The model under review builds one solid part; all positions refer to its coordinate system, in mm. A direction names the side the tool comes from. Round coordinates to 2 decimals unless told otherwise and drop trailing zeros. Write each loop counter-clockwise with the first axis right and the second up, starting at its lowest first coordinate (ties: lowest second). Pieces come first, ordered by that corner, then holes. Notation, with made-up numbers: (10.5, 74) - (63.5, 74) arc R24 cw to (63.5, 108) - close; hole circle Ø7 at (89, 46). An arc over 180 degrees is marked (long way). Write each question's results on one line, items separated by ' | '.
```python
from build123d import *

# Parameters (mm, degrees)
SKETCH1_R                 = 330.2
BOSS_EXTRUDE1_DEPTH       = 55
SKETCH2_R                 = 330.2
BOSS_EXTRUDE2_DEPTH       = 55
BOSS_EXTRUDE3_DEPTH       = 10
BOSS_EXTRUDE6_DEPTH       = 575.8
BOSS_EXTRUDE33_DEPTH      = 370
BOSS_EXTRUDE33_DEPTH_BACK = 370
SKETCH25_W                = 366.7
SKETCH25_H                = 80
SKETCH5_W                 = 450
SKETCH5_H                 = 72
BOSS_EXTRUDE7_DEPTH       = 367.981167426
SKETCH8_W                 = 49.2
SKETCH8_H                 = 29.2
BOSS_EXTRUDE13_DEPTH      = 30
SKETCH19_R                = 177.8
BOSS_EXTRUDE22_DEPTH      = 270.2
CHAMFER1_SIZE             = 100
CHAMFER1_SIZE2            = 93.251508614
BOSS_EXTRUDE27_DEPTH      = 30
BOSS_EXTRUDE20_DEPTH      = 260
SKETCH23_W                = 30
SKETCH23_H                = 60
SKETCH23_W_2              = 49.2
SKETCH23_H_2              = 25.4
SKETCH23_W_3              = 25.4
BOSS_EXTRUDE28_DEPTH      = 30
SKETCH24_R                = 177.8
BOSS_EXTRUDE29_DEPTH      = 270.2
CHAMFER2_SIZE             = 100
CHAMFER2_SIZE2            = 93.251508614
BOSS_EXTRUDE30_DEPTH      = 30
BOSS_EXTRUDE31_DEPTH      = 260
SKETCH16_W                = 250
SKETCH16_H                = 53.975
BOSS_EXTRUDE18_DEPTH      = 53.975
SKETCH18_W                = 250
SKETCH18_H                = 53.975
BOSS_EXTRUDE19_DEPTH      = 53.975
BOSS_EXTRUDE32_REACH      = 1866.083
BOSS_EXTRUDE34_REACH      = 1575.824
SKETCH26_W                = 154.1
SKETCH26_H                = 80
SKETCH27_W                = 350
SKETCH27_H                = 400
BOSS_EXTRUDE35_DEPTH      = 200
BOSS_EXTRUDE36_START      = -130
BOSS_EXTRUDE36_DEPTH      = 490
FILLET3_R                 = 50
SKETCH30_W                = 2623.123535912
SKETCH30_H                = 2390.43733062
CUT_EXTRUDE1_DEPTH        = 1887.551796433
SKETCH31_W                = 2584.765961417
SKETCH31_H                = 1828.147621016
CUT_EXTRUDE2_DEPTH        = 1855.050466041


with BuildPart() as part:
    # Sketch1 → Boss-Extrude1 (new body)
    with BuildSketch(Plane.XY):
        with Locations((330.2, 330.2)):
            Circle(SKETCH1_R)
    extrude(amount=-BOSS_EXTRUDE1_DEPTH)



with BuildPart() as body_2:
    # Sketch2 → Boss-Extrude2 (new body)
    with BuildSketch(Plane.XY.offset(-685.8)):
        with Locations((330.2, 330.2)):
            Circle(SKETCH2_R)
    extrude(amount=BOSS_EXTRUDE2_DEPTH)


with BuildPart() as part_1:
    add(part.part)

    add(body_2.part)  # Boss-Extrude3 merges body 2
    # 3DSketch2 → Boss-Extrude3 (add)
    with BuildSketch(Plane(origin=(330.2, 460, -630.8), x_dir=(0.5893057409504111, 0, 0.807910108664873), z_dir=(0, -1, 0))):
        Polygon((465.194640569, 339.322245639), (0, 0), (247.508411199, -339.322245639), (712.703051768, 0), align=None)
        Polygon((-38.304873162, 52.514157063), (0, 0), (465.194640569, 339.322245639), (426.889767407, 391.836402702), align=None)
    extrude(amount=-BOSS_EXTRUDE3_DEPTH)

    # Sketch4 → Boss-Extrude6 (add)
    with BuildSketch(Plane(origin=(0, -170.8, -630.8), x_dir=(1, 0, 0), z_dir=(0, 0, 1))):
        Polygon((208.828935151, 1364.6), (330.2, 501), (265.832575532, 491.953748438), (143.190142937, 1364.6), align=None)
    extrude(amount=BOSS_EXTRUDE6_DEPTH)

    # Sketch5 → Boss-Extrude7 (add, along a direction that is not the sketch's normal)
    with BuildSketch(Plane(origin=(0, 470, 0), x_dir=(1, 0, 0), z_dir=(0, 1, 0))):
        with Locations((535.552391309, 91)):
            Rectangle(SKETCH5_W, SKETCH5_H)
        with Locations((535.552391309, 594.8)):
            Rectangle(SKETCH5_W, SKETCH5_H)
    extrude(amount=BOSS_EXTRUDE7_DEPTH, dir=(-0.13917310096006222, 0.9902680687415708, 0))

    # Sketch8 → Boss-Extrude13 (add)
    with BuildSketch(Plane(origin=(0, 0, -630.8), x_dir=(-1, 0, 0), z_dir=(0, 0, -1))):
        Polygon((-1014.4, 360.2), (-939.8, 360.2), (-939.8, 330.2), (-914.4, 330.2), (-914.4, 270.2), (-884.4, 270.2), (-884.4, 330.2), (-330.2, 330.2), (-325.983774959, 360.2), (-914.4, 360.2), (-914.4, 414.8), (-884.4, 414.8), (-884.4, 440.2), (-1014.4, 440.2), align=None)
        with Locations((-964.4, 400.2)):
            Rectangle(SKETCH8_W, SKETCH8_H, mode=Mode.SUBTRACT)
    extrude(amount=-BOSS_EXTRUDE13_DEPTH)

    # Sketch19 → Boss-Extrude22 (add)
    with BuildSketch(Plane.XZ.offset(-270.2)):
        with Locations(Location((899.4, -615.8, 0), (0, 0, 90))):
            Circle(SKETCH19_R)
    extrude(amount=BOSS_EXTRUDE22_DEPTH)

    # Chamfer1
    chamfer1_edges = [part_1.edges().sort_by_distance(p)[0] for p in [
        (899.4, 270.2, -793.6),
    ]]
    chamfer1_side = [part_1.faces().sort_by_distance(p)[0] for p in [
        (899.4, 270.2, -788.571056572),
    ]]
    chamfer(chamfer1_edges, length=CHAMFER1_SIZE, length2=CHAMFER1_SIZE2, reference=chamfer1_side[0])

    # Sketch8<7> → Boss-Extrude27 (add)
    with BuildSketch(Plane(origin=(0, 0, -630.8), x_dir=(-1, 0, 0), z_dir=(0, 0, -1))):
        Polygon((-1014.4, 360.2), (-1140.7, 120.65), (-1115.3, 120.65), (-989, 360.2), align=None)
    extrude(amount=-BOSS_EXTRUDE27_DEPTH)

    # Sketch8<4> → Boss-Extrude20 (add)
    with BuildSketch(Plane(origin=(0, 0, -630.8), x_dir=(-1, 0, 0), z_dir=(0, 0, -1))):
        Polygon((-1226.425, 111.125), (-1226.425, 120.65), (-1140.7, 120.65), (-1115.3, 120.65), (-1029.575, 120.65), (-1029.575, 111.125), align=None)
    extrude(amount=-BOSS_EXTRUDE20_DEPTH)

    # Sketch23 → Boss-Extrude28 (add)
    with BuildSketch(Plane(origin=(0, 0, -55), x_dir=(-1, 0, 0), z_dir=(0, 0, -1))):
        with BuildLine():
            Line((-330.2, 360.2), (-659.034365601, 360.2))
            ThreePointArc((-659.034365601, 360.2), (-660.058414719, 345.215533268), (-660.4, 330.2))
            Line((-660.4, 330.2), (-330.2, 330.2))
            Line((-330.2, 330.2), (-330.2, 360.2))
        make_face()
        with BuildLine():
            Line((-914.4, 360.2), (-939.8, 360.2))
            Line((-939.8, 360.2), (-939.8, 330.2))
            Line((-939.8, 330.2), (-914.4, 330.2))
            Line((-914.4, 330.2), (-884.4, 330.2))
            Line((-884.4, 330.2), (-660.4, 330.2))
            ThreePointArc((-660.4, 330.2), (-660.058414719, 345.215533268), (-659.034365601, 360.2))
            Line((-659.034365601, 360.2), (-914.4, 360.2))
        make_face()
        with Locations((-899.4, 300.2)):
            Rectangle(SKETCH23_W, SKETCH23_H)
        Polygon((-939.8, 385.6), (-939.8, 360.2), (-914.4, 360.2), (-914.4, 414.8), (-914.4, 440.2), (-939.8, 440.2), (-939.8, 414.8), align=None)
        with Locations((-964.4, 372.9)):
            Rectangle(SKETCH23_W_2, SKETCH23_H_2)
        with Locations((-964.4, 427.5)):
            Rectangle(SKETCH23_W_2, SKETCH23_H_2)
        Polygon((-1014.4, 440.2), (-1014.4, 385.6), (-989, 385.6), (-989, 414.8), (-989, 440.2), align=None)
        with Locations((-1001.7, 372.9)):
            Rectangle(SKETCH23_W_3, SKETCH23_H_2)
        Polygon((-325.983774959, 360.2), (-330.2, 360.2), (-330.2, 330.2), align=None)
        with Locations((-899.4, 427.5)):
            Rectangle(SKETCH23_W, SKETCH23_H_2)
    extrude(amount=BOSS_EXTRUDE28_DEPTH)

    # Sketch24 → Boss-Extrude29 (add)
    with BuildSketch(Plane(origin=(0, 270.2, 0), x_dir=(-1, 0, 0), z_dir=(0, -1, 0))):
        with Locations(Location((-899.4, 70, 0), (0, 0, 270))):
            Circle(SKETCH24_R)
    extrude(amount=BOSS_EXTRUDE29_DEPTH)

    # Chamfer2
    chamfer2_edges = [part_1.edges().sort_by_distance(p)[0] for p in [
        (899.4, 270.2, -247.8),
    ]]
    chamfer2_side = [part_1.faces().sort_by_distance(p)[0] for p in [
        (899.4, 270.2, -242.771056572),
    ]]
    chamfer(chamfer2_edges, length=CHAMFER2_SIZE, length2=CHAMFER2_SIZE2, reference=chamfer2_side[0])

    # Sketch23<10> → Boss-Extrude30 (add)
    with BuildSketch(Plane(origin=(0, 0, -55), x_dir=(-1, 0, 0), z_dir=(0, 0, -1))):
        Polygon((-1014.4, 360.2), (-1140.7, 120.65), (-1115.3, 120.65), (-989, 360.2), align=None)
    extrude(amount=BOSS_EXTRUDE30_DEPTH)

    # Sketch23<12> → Boss-Extrude31 (add)
    with BuildSketch(Plane(origin=(0, 0, -55), x_dir=(-1, 0, 0), z_dir=(0, 0, -1))):
        Polygon((-1226.425, 111.125), (-1226.425, 120.65), (-1140.7, 120.65), (-1115.3, 120.65), (-1029.575, 120.65), (-1029.575, 111.125), align=None)
    extrude(amount=BOSS_EXTRUDE31_DEPTH)

    # Sketch16 → Boss-Extrude18 (add)
    with BuildSketch(Plane(origin=(0, 0, -630.8), x_dir=(-1, 0, 0), z_dir=(0, 0, -1))):
        with Locations((-58.349686454, 935.0375)):
            Rectangle(SKETCH16_W, SKETCH16_H)
    extrude(amount=-BOSS_EXTRUDE18_DEPTH)

    # Sketch18 → Boss-Extrude19 (add)
    with BuildSketch(Plane(origin=(0, 0, -55), x_dir=(-1, 0, 0), z_dir=(0, 0, -1))):
        with Locations((-58.349686454, 935.0375)):
            Rectangle(SKETCH18_W, SKETCH18_H)
    extrude(amount=BOSS_EXTRUDE19_DEPTH)

    # Boss-Extrude32: up to this face of the body (flat: up to its plane)
    boss_extrude32_end = Plane(part_1.part.faces().sort_by_distance((283.205191665, 255.458003874, -55))[0])
    # Sketch8<8> → Boss-Extrude32 (add, up to the picked face)
    with BuildSketch(Plane(origin=(0, 0, -630.8), x_dir=(-1, 0, 0), z_dir=(0, 0, -1)), mode=Mode.PRIVATE) as boss_extrude32_sk1:
        Polygon((-314.740508183, 440.2), (-283.793416381, 660.4), (-914.4, 660.4), (-914.4, 440.2), align=None)
    boss_extrude32_tool1 = split(extrude(boss_extrude32_sk1.sketch, amount=-BOSS_EXTRUDE32_REACH, mode=Mode.PRIVATE), bisect_by=boss_extrude32_end, keep=Keep.BOTH, mode=Mode.PRIVATE)
    add(boss_extrude32_tool1.solids().sort_by(Axis((606.768609, 551.223181, -630.8), (0, 0, 1)))[0])



with BuildPart() as body_2_2:
    # Sketch25 → Boss-Extrude33 (new, two sides: drawn at the far end of the back side and taken through both)
    with BuildSketch(Plane.XY.offset(-342.9).offset(-BOSS_EXTRUDE33_DEPTH_BACK)):
        with Locations((760.189311143, 874.4)):
            Rectangle(SKETCH25_W, SKETCH25_H)
    extrude(amount=BOSS_EXTRUDE33_DEPTH + BOSS_EXTRUDE33_DEPTH_BACK)


with BuildPart() as part_2:
    add(part_1.part)

    add(body_2_2.part)  # Boss-Extrude34 merges body 2 2
    # Boss-Extrude34: up to this plane
    boss_extrude34_end = Plane(origin=(143.190142937, 1193.8, 837.459616456), z_dir=(0.9902680687415708, 0.13917310096006216, 0))
    # Sketch26 → Boss-Extrude34 (add, up to the surface)
    with BuildSketch(Plane.ZY.offset(-576.839311143), mode=Mode.PRIVATE) as boss_extrude34_sk1:
        with Locations((-49.95, 874.4)):
            Rectangle(SKETCH26_W, SKETCH26_H)
    boss_extrude34_tool1 = split(extrude(boss_extrude34_sk1.sketch, amount=BOSS_EXTRUDE34_REACH, mode=Mode.PRIVATE), bisect_by=boss_extrude34_end, keep=Keep.BOTH, mode=Mode.PRIVATE)
    add(boss_extrude34_tool1.solids().sort_by_distance((576.839311, 874.4, -49.95))[0])
    # Sketch26 → Boss-Extrude34 (add, up to the surface)
    with BuildSketch(Plane.ZY.offset(-576.839311143), mode=Mode.PRIVATE) as boss_extrude34_sk2:
        with Locations((-635.85, 874.4)):
            Rectangle(SKETCH26_W, SKETCH26_H)
    boss_extrude34_tool2 = split(extrude(boss_extrude34_sk2.sketch, amount=BOSS_EXTRUDE34_REACH, mode=Mode.PRIVATE), bisect_by=boss_extrude34_end, keep=Keep.BOTH, mode=Mode.PRIVATE)
    add(boss_extrude34_tool2.solids().sort_by_distance((576.839311, 874.4, -635.85))[0])

    # Sketch27 → Boss-Extrude35 (add)
    with BuildSketch(Plane(origin=(304.944608977, 42.857169884, 0), x_dir=(0, 0, 1), z_dir=(-0.9902680687415708, -0.13917310096006216, 0))):
        with Locations((-342.9, 481.031558361)):
            Rectangle(SKETCH27_W, SKETCH27_H)
    extrude(amount=BOSS_EXTRUDE35_DEPTH)

    # Sketch29 → Boss-Extrude36 (add)
    with BuildSketch(Plane(origin=(0, 0, -712.9), x_dir=(-1, 0, 0), z_dir=(0, 0, -1)).offset(BOSS_EXTRUDE36_START)):
        Polygon((-1029.044346974, 1149.323155196), (-986.95135556, 1160.601938253), (-943.539311143, 914.4), align=None)
        Polygon((-986.95135556, 1160.601938253), (-943.539311143, 914.4), (-923.230778905, 914.4), (-967.2552005, 1164.074901806), align=None)
    extrude(amount=-BOSS_EXTRUDE36_DEPTH)

    # Fillet3
    fillet3_edges = [part_2.edges().sort_by_distance(p)[0] for p in [
        (914.4, 660.4, -342.9),
    ]]
    fillet(fillet3_edges, radius=FILLET3_R)

    # Sketch30 → Cut-Extrude1 (cut, through all)
    with BuildSketch(Plane.XY):
        with Locations((451.826678709, -534.81866531)):
            Rectangle(SKETCH30_W, SKETCH30_H)
    extrude(amount=CUT_EXTRUDE1_DEPTH, mode=Mode.SUBTRACT)

    # Sketch31 → Cut-Extrude2 (cut, through all)
    with BuildSketch(Plane(origin=(0, 0, -685.8), x_dir=(-1, 0, 0), z_dir=(0, 0, -1))):
        with Locations((-741.050727566, -253.673810508)):
            Rectangle(SKETCH31_W, SKETCH31_H)
    extrude(amount=CUT_EXTRUDE2_DEPTH, mode=Mode.SUBTRACT)


solid = part_2.part
```
Q1. The part is to be moulded in two halves that separate along Z. For faces 5 (the flat face through (964, 440.2, -616)), 6 (the flat face through (975, 1069, -582.9)), 7 (the flat face through (826, 340, -600.8)), say which applies: released by +Z, released by -Z, zero draft, split by the parting line, or undercut.
Evaluation:
face 5: zero draft | face 6: released by -Z | face 7: undercut
Q2. We need section B-B (y = 547). State the section outline as (x, z) points, plus the area to 3 significant figures.
Evaluation:
outline: (32.13, -517.9) - (234.09, -517.9) - (234.09, -630.8) - (81.14, -630.8) - (81.14, -685.8) - (579.26, -685.8) - (579.26, -630.8) - (914.4, -630.8) - (914.4, -55) - (579.26, -55) - (579.26, 0) - (81.14, 0) - (81.14, -55) - (234.09, -55) - (234.09, -167.9) - (32.13, -167.9) - close | area: 517,000 mm^2
Q3. Tool access review of faces 1 (the flat face through (914.4, 526, -347)), 2 (the flat face through (939.8, 345, -70)), 3 (the flat face through (60, 908.05, -82)), 4 (the flat face through (494, 786, -127)): name each direction out of +Z, -Z, +X, -X, +Y, -Y from which nothing blocks a thin tool from reaching the whole face with its end or side.
Evaluation:
face 1: +Z, -Z, +X | face 2: +Z, -Z | face 3: +Z, -Z, -X, -Y | face 4: none
Q4. Insertion check: P1, Ø4, axis at x = 256.5, y = 746.5, coming from the +Z side; P2, Ø9, axis at x = 627.5, z = -610.5, coming from the +Y side; P3, Ø15, axis at y = 340, z = -65.5, coming from the +X side. Each pin has a flat end and moves straight along its axis. Give the tip position at first contact, or say it passes through.
Evaluation:
P1: stops at z = -55 | P2: stops at y = 914.4 | P3: stops at x = 1029
Q5. For probe 1 along Y at (x, z) = (851.5, -609); probe 2 along Z at (x, y) = (197.5, 478); probe 3 along Y at (x, z) = (597, -513), list the stretches that pass through material, from the lowest coordinate up.
Evaluation:
probe 1: y = 0 to 270.2, 330.2 to 360.2, 440.2 to 660.4, 834.4 to 914.4 | probe 2: z = -685.8 to -630.8, -517.9 to -167.9, -55 to 0 | probe 3: y = 440.2 to 660.4, 834.4 to 914.4
Q6. We need section A-A (x = 451.5). State the section outline as (y, z) points.
Evaluation:
outline: (23.09, -685.8) - (637.31, -685.8) - (637.31, -630.8) - (834.4, -630.8) - (834.4, -712.9) - (914.4, -712.9) - (914.4, -558.8) - (660.4, -558.8) - (660.4, -127) - (914.4, -127) - (914.4, 27.1) - (834.4, 27.1) - (834.4, -55) - (637.31, -55) - (637.31, 0) - (23.09, 0) - (23.09, -55) - (330.2, -55) - (330.2, -85) - (360.2, -85) - (360.2, -55) - (440.2, -55) - (440.2, -630.8) - (360.2, -630.8) - (360.2, -600.8) - (330.2, -600.8) - (330.2, -630.8) - (23.09, -630.8) - close
